Could you check a few things on this drawing? It's one solid part, dimensions in mm from its lowest x, y, z. A direction names the side the tool comes from. Give positions to 0.01 mm unless a question says otherwise; leave off trailing zeros. Loops run counter-clockwise (first coordinate to the right, second up) from the corner with the lowest first, then second, coordinate; pieces in that order, holes last. Notation, with made-up numbers: (71.25, 7.5) - (78.25, 7.5) arc R21 cw to (78.25, 36.5) - close; hole circle Ø4 at (-35, 82). An arc over 180 degrees is marked (long way). Use a Markdown table: item, result.
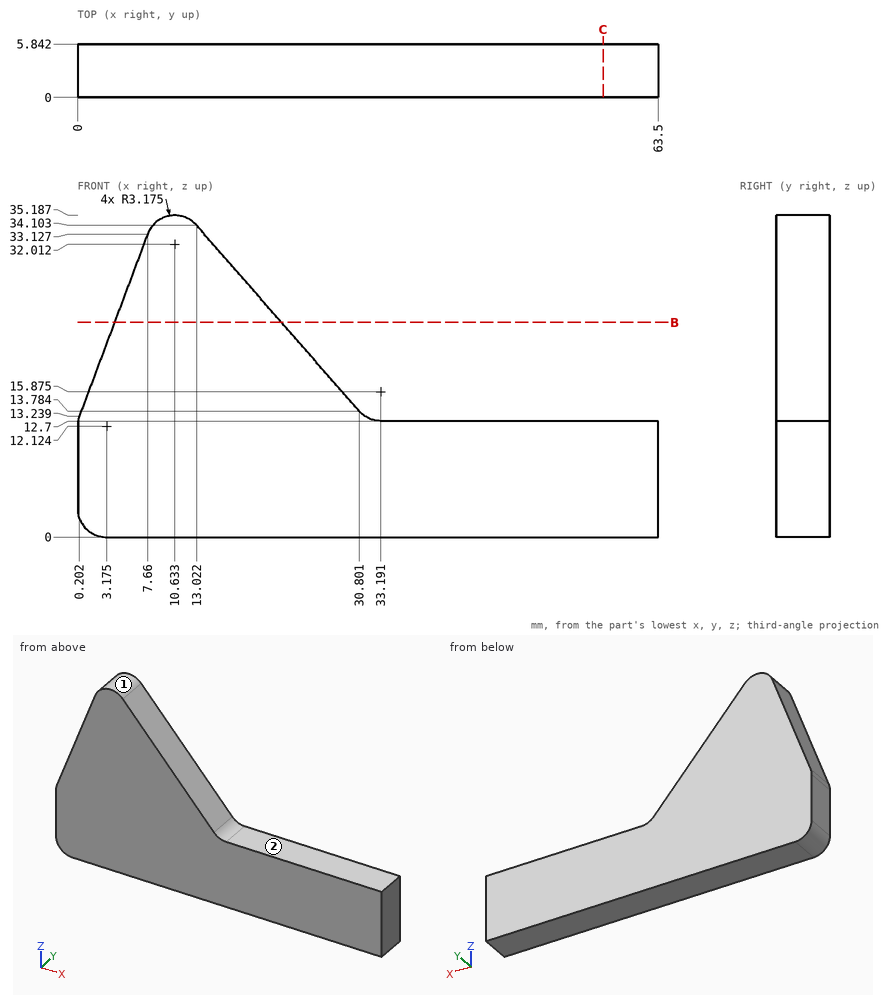
(1) Suppose I cut it at C-C on x = 57.5. Write out the boundary of the cut face in (y, z), plus the area to 3 significant figures.
A:
| item | result |
|---|---|
| outline | (0, 0) - (5.84, 0) - (5.84, 12.7) - (0, 12.7) - close |
| area | 74.2 mm2 |
(2) Will these pins go through, and if not, where does the flat tip stop? pin 1 (3 mm diameter, centred on y = 5, z = 16, fed in from +X) (1 decimal); pin 2 (2 mm diameter, centred on y = 1.5, z = 18.5, fed in from -X).
A:
| item | result |
|---|---|
| pin 1 | x = 30.2 |
| pin 2 | x = 1.8 |
(3) Suppose I cut it at B-B on z = 23.5. Write out the boundary of the cut face in (x, y).
A:
| item | result |
|---|---|
| outline | (4.05, 0) - (22.3, 0) - (22.3, 5.84) - (4.05, 5.84) - close |
(4) If I drill on line 1 (Z direction, x = 36, y = 1.9); line 2 (X direction, y = 3.7, z = 3) (1 decimal); line 3 (Z direction, x = 32.5, y = 5.1) (1 decimal), over which ranges is the centre line in solid material (lowest first)?
A:
| item | result |
|---|---|
| line 1 | 0 to 12.7 |
| line 2 | 0 to 63.5 |
| line 3 | 0 to 12.8 |
(5) On a 3-axis mill with a long thin cutter (end or side, diameter ignored), from which of +Z, -Z, +X, -X, +Y, -Y can I reach the whole of each face in a straight line? I mean the marked faces 1 and 2. Say none if no direction works.
A:
| item | result |
|---|---|
| face 1 | +Z, +Y, -Y |
| face 2 | +Z, +X, +Y, -Y |
